The model under review builds one solid part; all positions refer to its coordinate system, in mm. A direction names the side the tool comes from. Round coordinates to 2 decimals unless told otherwise and drop trailing zeros. Write each loop counter-clockwise with the first axis right and the second up, starting at its lowest first coordinate (ties: lowest second). Pieces come first, ordered by that corner, then holes.
Item 1: Clearance check with flat-ended pins moving along their axes: pin 1 Ø1.5 at (x, y) = (0.5, 28) entering from +Z; pin 2 Ø3 at (y, z) = (5, 0) entering from -X; pin 3 Ø2 at (x, z) = (1.5, -1.5) entering from +Y. State where each tip first meets the part, or that it passes through.
Item 2: Add section D-D (x = 1.15). Give the boundary of the cut face in (y, z).
Item 3: Draft analysis for pull direction Z (two halves, no side actions). For faces 4 (the face through (-0.028, 14.524, 0.632)), 5 (the face through (0, 12, -4)), 6 (the face through (1, 20, 0)), 7 (the face through (-1, 32, 0.5)), state which applies: +Z half, -Z half, draft (parallel to the pull), parting line (faces both ways), or undercut.
Item 4: To check wall thickness, follow L1, parallel to Z at x = 0.25, y = 13; L2, parallel to Y at x = -0.45, z = -1.5; L3, parallel to Y at x = 0.45, z = -1.5. State the ranges of each line that lie inside material, in increasing order.
Item 5: Add section C-C (x = -1). Give the boundary of the cut face in (y, z).
Item 6: Machinability: for faces 1 (the face through (-1.01, 34.1, 3.14)), 2 (the face through (0, 27, 0)), 3 (the face through (-1, 34, 0)), which of the approach directions +Z, -Z, +X, -X, +Y, -Y give a long, thin tool a straight path to every point of the face, cutting with its end or side? Answer none if there is none.
Item 7: Add section A-A (z = 0). Give the boundary of the cut face in (x, y), plus the area to 3 significant figures.
Item 8: Add section B-B (y = 13). Give the boundary of the cut face in (x, z), plus the area to 3 significant figures.
Autodesk Inventor part; units mm, degrees
ref_plane "YZ Plane" through (0, 0, 0) normal (1, 0, 0) x (0, 1, 0)
ref_plane "XZ Plane" through (0, 0, 0) normal (0, 1, 0) x (-1, 0, 0)
ref_plane "XY Plane" through (0, 0, 0) normal (0, 0, 1) x (1, 0, 0)
sketch "Sketch1" plane through (0, 0, 0) normal (1, 0, 0) x (0, 1, 0)
  line L0 (35, 4) -> (0, 4)
  line L1 (0, 4) -> (0, -4)
  line L2 (0, -4) -> (35, -4)
  line L3 (35, -4) -> (35, 4)
  line L4 (34, 0.5) -> (29, 0.5)
  line L5 (29, 0.5) -> (29, -0.5)
  line L6 (29, -0.5) -> (34, -0.5)
  line L7 (34, -0.5) -> (34, 0.5)
  line L8 (20, 4) -> (20, -4)
  circle A0 centre (13, 0) radius 1.65
  circle A1 centre (5, 0) radius 1.65
  point P0 (0, 0)
  point P1 (0, 0)
  point P2 (29, 0)
  point P3 (20, 0)
  dimension "d0" = 8
  dimension "d2" = 1
  dimension "d3" = 1
  dimension "d4" = 5
  dimension "d5" = 20
  dimension "d6" = 15
  dimension "d7" = 3.3
  dimension "d8" = 3.3
  dimension "d9" = 7
  dimension "d10" = 8
extrude "Extrusion1" add sketch "Sketch1" along normal blind 2 contours L8 L2 L1 L0
extrude "Extrusion2" add sketch "Sketch1" against normal blind 2
fillet "Fillet1" radius 3 2 edges at (-1, 35, 4) (-1, 35, -4)
properties part number "MUESCA_DETECCION_CERO" material "Steel, Mild, Welded"
Numbers:
1. pin 1: stops at z = 4
1. pin 2: passes through
1. pin 3: stops at y = 20
2. outline: (0, -4) - (20, -4) - (20, 4) - (0, 4) - close; hole circle Ø3.3 at (5, 0); hole circle Ø3.3 at (13, 0)
3. face 4: undercut
3. face 5: -Z half
3. face 6: draft
3. face 7: undercut
4. L1: z = -4 to -1.65, 1.65 to 4
4. L2: y = 0 to 4.31, 5.69 to 12.31, 13.69 to 34.96
4. L3: y = 0 to 4.31, 5.69 to 12.31, 13.69 to 20
5. outline: (0, -4) - (32, -4) arc R3 ccw to (35, -1) - (35, 1) arc R3 ccw to (32, 4) - (0, 4) - close; hole circle Ø3.3 at (5, 0); hole circle Ø3.3 at (13, 0); hole (29, -0.5) - (34, -0.5) - (34, 0.5) - (29, 0.5) - close
6. face 1: +Z, +X, -X, +Y
6. face 2: +Z, -Z, +X, +Y
6. face 3: +X, -X
7. outline: (-2, 0) - (2, 0) - (2, 3.35) - (-2, 3.35) - close; (-2, 6.65) - (2, 6.65) - (2, 11.35) - (-2, 11.35) - close; (-2, 14.65) - (2, 14.65) - (2, 20) - (0, 20) - (0, 29) - (-2, 29) - close; (-2, 34) - (0, 34) - (0, 35) - (-2, 35) - close
7. area: 73.6 mm2
8. outline: (-2, -4) - (2, -4) - (2, -1.65) - (-2, -1.65) - close; (-2, 1.65) - (2, 1.65) - (2, 4) - (-2, 4) - close
8. area: 18.8 mm2
